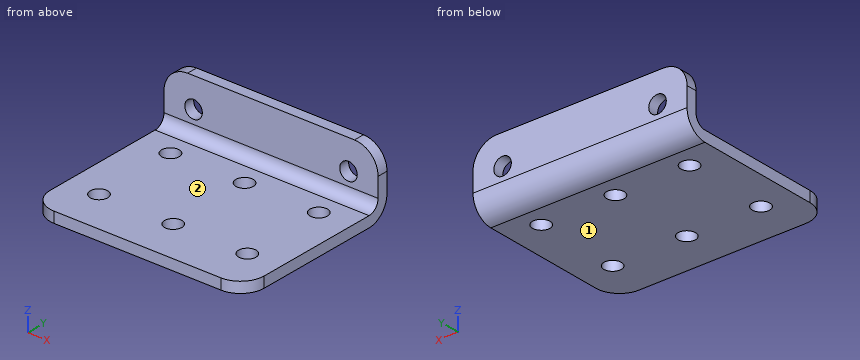
from build123d import *

# Parameters (mm, degrees)
SKETCH2_W              = 63.5
SKETCH2_H              = 50.679996867
BOSS_EXTRUDE1_DEPTH    = 3.175
SKETCH3_W              = 63.5
SKETCH3_H              = 19.05
BOSS_EXTRUDE2_DEPTH    = 3.175
SKETCH4_R              = 2.6
CUT_EXTRUDE1_DEPTH     = 3.175
FILLET1_R              = 7
CONVERT_SOLID1_START   = -457.2
CONVERT_SOLID1_DEPTH   = 63.5
CONVERT_SOLID1_2_DEPTH = 63.5
SKETCH5_R              = 2.6
CUT_EXTRUDE2_DEPTH     = 10


# Read off the part's stored shape, not the designer's step: Convert-Solid1
with BuildPart() as part:
    # Sketch2 → Boss-Extrude1 (new body)
    with BuildSketch(Plane.XY):
        with Locations((-425.45, -0.060001567)):
            Rectangle(SKETCH2_W, SKETCH2_H)
    extrude(amount=BOSS_EXTRUDE1_DEPTH)

    # Sketch3 → Boss-Extrude2 (add)
    with BuildSketch(Plane(origin=(0, 25.279996867, 0), x_dir=(1, 0, 0), z_dir=(0, 1, 0))):
        with Locations((-425.45, -9.525)):
            Rectangle(SKETCH3_W, SKETCH3_H)
    extrude(amount=-BOSS_EXTRUDE2_DEPTH)

    # Sketch4 → Cut-Extrude1 (cut)
    with BuildSketch(Plane.XZ.offset(-22.104996867)):
        with Locations((-402.469029611, 10.280970389)):
            Circle(SKETCH4_R)
        with Locations((-448.430970389, 10.280970389)):
            Circle(SKETCH4_R)
    extrude(amount=-CUT_EXTRUDE1_DEPTH, mode=Mode.SUBTRACT)

    # Fillet1
    fillet1_edges = [part.edges().sort_by_distance(p)[0] for p in [
        (-457.2, 23.692496867, 19.05),
        (-393.7, 23.692496867, 19.05),
        (-393.7, -25.4, 1.5875),
        (-457.2, -25.4, 1.5875),
    ]]
    fillet(fillet1_edges, radius=FILLET1_R)

    # Convert-Solid1 outline → Convert-Solid1 (cut)
    with BuildSketch(Plane.YZ.offset(CONVERT_SOLID1_START)):
        with BuildLine():
            Line((25.279996867, 0), (25.279996867, 6.35))
            ThreePointArc((25.279996867, 6.35), (23.420124928, 1.859871939), (18.929996867, 0))
            Line((18.929996867, 0), (25.279996867, 0))
        make_face()
    extrude(amount=CONVERT_SOLID1_DEPTH, mode=Mode.SUBTRACT)

    # Convert-Solid1 2 outline → Convert-Solid1 2 (add)
    with BuildSketch(Plane.YZ.offset(CONVERT_SOLID1_START)):
        with BuildLine():
            Line((22.104996867, 3.175), (22.104996867, 6.35))
            ThreePointArc((22.104996867, 6.35), (21.175060897, 4.10493597), (18.929996867, 3.175))
            Line((18.929996867, 3.175), (22.104996867, 3.175))
        make_face()
    extrude(amount=CONVERT_SOLID1_2_DEPTH)

    # Sketch5 → Cut-Extrude2 (cut)
    with BuildSketch(Plane.XY.offset(3.175)):
        with Locations((-447.45, 12.7)):
            Circle(SKETCH5_R)
        with Locations((-425.45, 12.7)):
            Circle(SKETCH5_R)
        with Locations((-403.45, 12.7)):
            Circle(SKETCH5_R)
        with Locations((-403.45, -12.7)):
            Circle(SKETCH5_R)
        with Locations((-425.45, -12.7)):
            Circle(SKETCH5_R)
        with Locations((-447.45, -12.7)):
            Circle(SKETCH5_R)
    extrude(amount=-CUT_EXTRUDE2_DEPTH, mode=Mode.SUBTRACT)


solid = part.part
Work out the finished part from the listing and answer in its coordinate system (mm). Face numbers are marked on the shaded views. A direction names the side the tool comes from. Round coordinates to 2 decimals unless told otherwise and drop trailing zeros. Order: outer loops, then holes, each group sorted by start corner. A loop starts at its lowest first (then second) coordinate and runs counter-clockwise, first axis right, second up. Notation, with made-up numbers: M 11.25,-25 L 63.25,-25 A21 ccw 63.25,10 Z; hole C 22,27.5 d7. An arc over 180 degrees is marked long. One line per item, written item: value.
Q1. Find section C-C on x = -403.45. Write down the section's boundary in (y, z) (3 decimals), then the cut area to 3 significant figures.
Derived:
outline: M -25.4,0 L -15.3,0 L -15.3,3.175 L -25.4,3.175 Z; M -10.1,0 L 10.1,0 L 10.1,3.175 L -10.1,3.175 Z; M 15.3,0 L 18.93,0 A6.35 ccw 25.28,6.35 L 25.28,7.873 L 22.105,7.873 L 22.105,6.35 A3.175 cw 18.93,3.175 L 15.3,3.175 Z; M 22.105,12.689 L 25.28,12.689 L 25.28,19.05 L 22.105,19.05 Z
area: 157 mm²
Q2. Find section A-A on y = -12.7. Write down the section's boundary in (x, z) (3 decimals).
Derived:
outline: M -457.2,0 L -450.05,0 L -450.05,3.175 L -457.2,3.175 Z; M -444.85,0 L -428.05,0 L -428.05,3.175 L -444.85,3.175 Z; M -422.85,0 L -406.05,0 L -406.05,3.175 L -422.85,3.175 Z; M -400.85,0 L -393.7,0 L -393.7,3.175 L -400.85,3.175 Z
Q3. Straight lines are drawn through the part: line 1 (Y direction, x = -447.45, z = 1.8); line 2 (Z direction, x = -405, y = -15) (3 decimals); line 3 (X direction, y = -15, z = 1.75). For each, find the intervals that lie inside material, in ascending order.
Derived:
line 1: -25.4 to -15.3, -10.1 to 10.1, 15.3 to 23.36
line 2: 0 to 3.175
line 3: -457.2 to -448.66, -446.24 to -426.66, -424.24 to -404.66, -402.24 to -393.7
Q4. Find section D-D on z = 8.5. Write down the section's boundary in (x, y) (3 decimals), then the cut area to 3 significant figures.
Derived:
outline: M -457.2,22.105 L -450.325,22.105 L -450.325,25.28 L -457.2,25.28 Z; M -446.537,22.105 L -404.363,22.105 L -404.363,25.28 L -446.537,25.28 Z; M -400.575,22.105 L -393.7,22.105 L -393.7,25.28 L -400.575,25.28 Z
area: 178 mm²
Q5. For the marked faces 1 and 2, determine the directions among +Z, -Z, +X, -X, +Y, -Y from which every point of the face is accessible in a straight line to the end or side of a thin tool.
Derived:
face 1: -Z, +X, -X, +Y, -Y
face 2: +Z, +X, -X, -Y
Q6. Find section B-B on x = -425.45. Write down the section's boundary in (y, z) (3 decimals), then the cut area to 3 significant figures.
Derived:
outline: M -25.4,0 L -15.3,0 L -15.3,3.175 L -25.4,3.175 Z; M -10.1,0 L 10.1,0 L 10.1,3.175 L -10.1,3.175 Z; M 15.3,0 L 18.93,0 A6.35 ccw 25.28,6.35 L 25.28,19.05 L 22.105,19.05 L 22.105,6.35 A3.175 cw 18.93,3.175 L 15.3,3.175 Z
area: 172 mm²
Q7. Flat-ended cylindrical pins translate along their axes: pin 1 (3 mm diameter, centred on x = -448.43, z = 10.28, fed in from +Y); pin 2 (6 mm diameter, centred on x = -435, y = -17.5, fed in from +Z) (3 decimals); pin 3 (1 mm diameter, centred on x = -420, z = 15.5, fed in from -Y) (3 decimals). Find the tip coordinate at first contact, or state that the pin passes through.
Derived:
pin 1: through
pin 2: z = 3.175
pin 3: y = 22.105
